Geometry check sheet. Reference: drawing and pictorial views, mm from the part's lowest x, y, z. Give positions to 0.01 mm unless a question says otherwise; leave off trailing zeros. Write each loop counter-clockwise with the first axis right and the second up, starting at its lowest first coordinate (ties: lowest second). Pieces come first, ordered by that corner, then holes. Notation, with made-up numbers: M 20.5,69.5 L 40.5,69.5 A5 ccw 40.5,74.5 Z; hole C 13.5,71.25 d7. An arc over 180 degrees is marked long. Write each question's results on one line, items separated by ' | '. Start each with the question number.
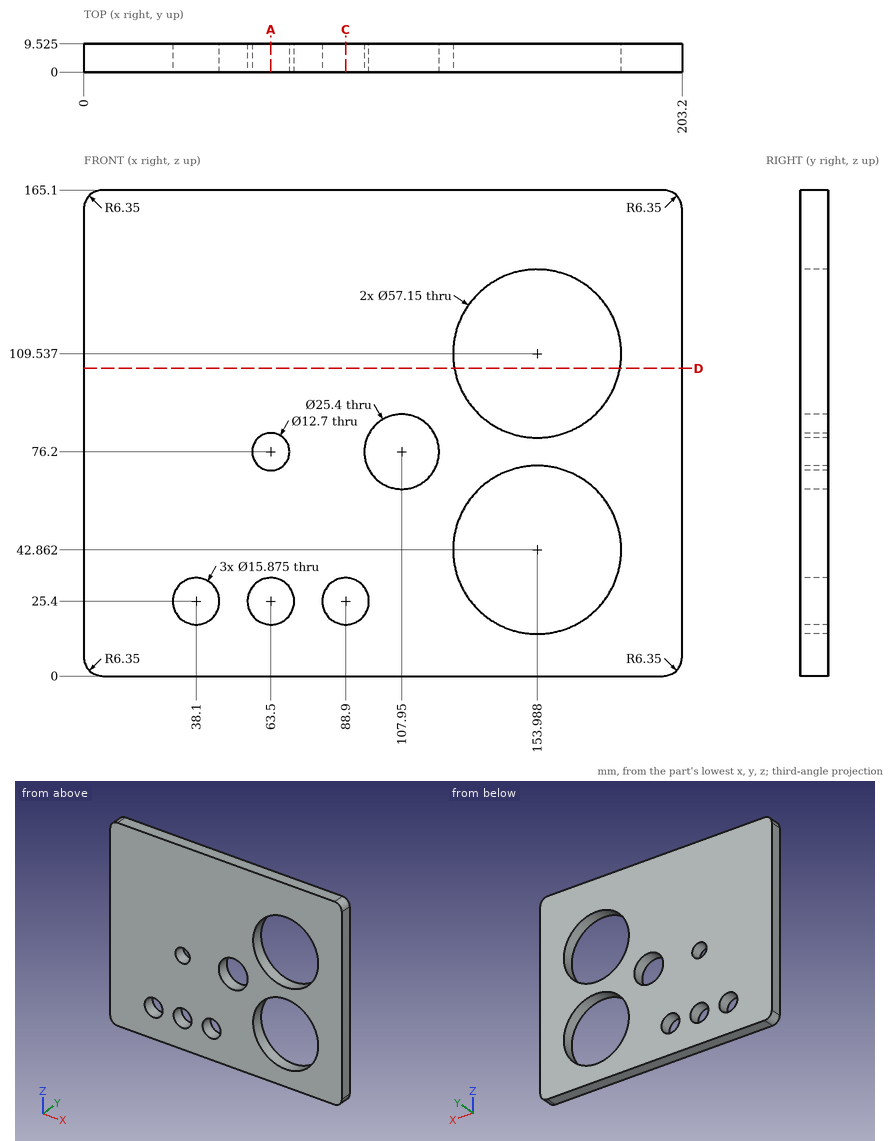
Q1. Scan lines: L1, parallel to Z at x = 63.5, y = 5; L2, parallel to Z at x = 169.5, y = 4.5 (1 decimal); L3, parallel to X at y = 6.5, z = 116. Record each from-to range of solid material in increasing order.
Q2. Section check D-D on z = 104.5. Record the boundary of the cut face in (x, y) (1 decimal), plus the area to 3 significant figures.
Q3. Section check C-C on x = 88.9. Record the boundary of the cut face in (y, z) (1 decimal), plus the area to 3 significant figures.
Q4. Depth check by flat-ended pin: pin 1 Ø6 at (x, z) = (157, 73.5) entering from -Y; pin 2 Ø20.5 at (x, z) = (107.95, 76.2) entering from -Y. Enter the tip coordinate at first touch or a pass-through.
Q5. Section check A-A on x = 63.5. State how many separate pieces and enclosed holes the cut face has, plus the area to 3 significant figures.
Check result:
1) L1: 0 to 17.46, 33.34 to 69.85, 82.55 to 165.1 | L2: 0 to 18.9, 66.9 to 85.5, 133.5 to 165.1 | L3: 0 to 126.15, 181.82 to 203.2
2) outline: M 0,0 L 125.9,0 L 125.9,9.5 L 0,9.5 Z; M 182.1,0 L 203.2,0 L 203.2,9.5 L 182.1,9.5 Z | area: 1,400 mm^2
3) outline: M 0,0 L 9.5,0 L 9.5,17.5 L 0,17.5 Z; M 0,33.3 L 9.5,33.3 L 9.5,165.1 L 0,165.1 Z | area: 1,420 mm^2
4) pin 1: y = 0 | pin 2: through
5) separate pieces: 3 | enclosed holes: 0 | area: 1,300 mm^2
